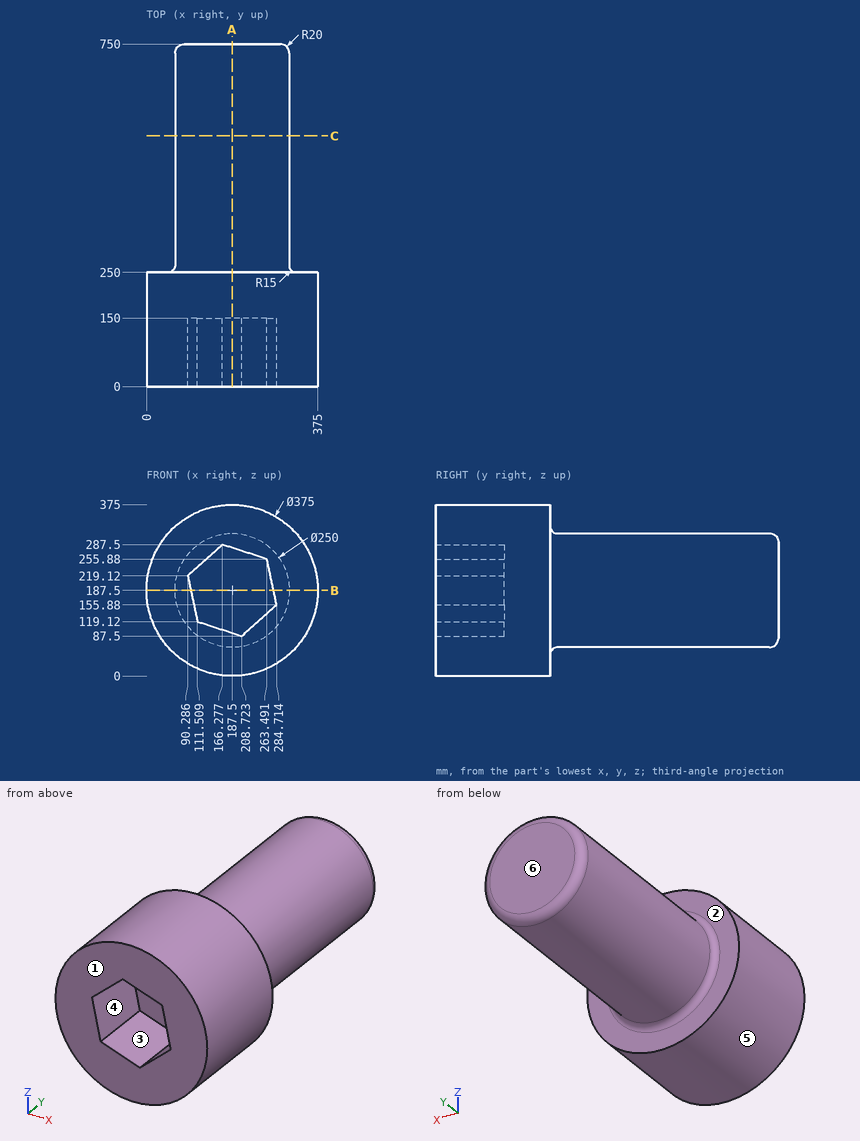
Source: three-view drawing plus pictorial views. Frame: mm from the lowest corner of the part. A direction names the side the tool comes from. Give positions to 0.01 mm unless a question says otherwise; leave off trailing zeros. Order: outer loops, then holes, each group sorted by start corner. A loop starts at its lowest first (then second) coordinate and runs counter-clockwise, first axis right, second up. Notation, with made-up numbers: (-0.5, 53.25) -> (46.5, 53.25) arc R28 cw to (46.5, 87.25) -> close; hole circle Ø10 at (-13, -18.5). An arc over 180 degrees is marked (long way). Write each question's results on one line, items separated by ' | '. Start each with the question number.
Item 1: Contact query for flat-ended pins moving along their axis: P1, Ø10, axis at x = 231, y = 356, coming from the -Z side; P2, Ø3, axis at x = 136, y = 129.5, coming from the -Z side; P3, Ø1.5, axis at x = 126.5, y = 407.5, coming from the -Z side. Output: stop coordinate, or through.
Item 2: Set-up query: the marked faces 1, 2 and 3. Return all of +Z, -Z, +X, -X, +Y, -Y with unobstructed straight access to the full face (end or side cutting, diameter ignored); none if empty.
Item 3: Cut plane A-A on x = 187.5. Return the cut outline in (y, z), then the cut area to 3 significant figures.
Item 4: Cut plane B-B on z = 187.5. Return the cut outline in (x, y), then the cut area to 3 significant figures.
Item 5: Line query: line 1 (Y direction, x = 120.5, z = 318.5); line 2 (Z direction, x = 256, y = 75) (1 decimal); line 3 (Y direction, x = 217, z = 128). Output: solid intervals per line, ascending.
Item 6: Mould query, pull axis Z, two halves, no side actions, for the marked faces 4, 5 and 6. Classes: pulls with the +Z half, pulls with the -Z half, needs draft (parallel to the pull), parting line crosses it, or undercut.
Item 7: Cut plane C-C on y = 549. Return the cut outline in (x, z), then the cut area to 3 significant figures.
Established:
1) P1: z = 68.58 | P2: z = 6.79 | P3: z = 77.98
2) face 1: +Z, -Z, +X, -X, -Y | face 2: +Y | face 3: -Y
3) outline: (0, 0) -> (250, 0) -> (250, 47.5) arc R15 cw to (265, 62.5) -> (730, 62.5) arc R20 ccw to (750, 82.5) -> (750, 292.5) arc R20 ccw to (730, 312.5) -> (265, 312.5) arc R15 cw to (250, 327.5) -> (250, 375) -> (0, 375) -> (0, 280.6) -> (150, 280.6) -> (150, 94.4) -> (0, 94.4) -> close | area: 191,000 mm^2
4) outline: (0, 0) -> (97, 0) -> (97, 150) -> (278, 150) -> (278, 0) -> (375, 0) -> (375, 250) -> (327.5, 250) arc R15 cw to (312.5, 265) -> (312.5, 730) arc R20 ccw to (292.5, 750) -> (82.5, 750) arc R20 ccw to (62.5, 730) -> (62.5, 265) arc R15 cw to (47.5, 250) -> (0, 250) -> close | area: 192,000 mm^2
5) line 1: 0 to 250 | line 2: 13 to 130, 258.3 to 362 | line 3: 150 to 750
6) face 4: undercut | face 5: parting line crosses it | face 6: needs draft
7) outline: circle Ø250 at (187.5, 187.5) | area: 49,100 mm^2
